```python
from build123d import *

# Parameters (mm, degrees)
DODANIE_WYCI_GNI_CIE1_DEPTH     = 3
SZKIC2_R                        = 1.35
WYTNIJ_WYCI_GNI_CIE1_DEPTH      = 3
DODANIE_WYCI_GNI_CIE2_DEPTH     = 40
WYTNIJ_WYCI_GNI_CIE4_DEPTH      = 65.691575959
WYTNIJ_WYCI_GNI_CIE4_DEPTH_BACK = 65.691575959
SZKIC6_R                        = 1.05
ZAOKR_GLENIE8_R                 = 20
ZAOKR_GLENIE9_R                 = 20
ZAOKR_GLENIE10_R                = 2
ZAOKR_GLENIE11_R                = 2


with BuildPart() as part:
    # Szkic1 → Dodanie-wyciągnięcie1 (new body)
    with BuildSketch(Plane(origin=(0, 0, 0), x_dir=(1, 0, 0), z_dir=(0, 1, 0))):
        with BuildLine():
            Line((-23.5, -20), (23.5, -20))
            ThreePointArc((23.5, -20), (24.560660172, -19.560660172), (25, -18.5))
            Line((25, -18.5), (25, 18.5))
            ThreePointArc((25, 18.5), (24.560660172, 19.560660172), (23.5, 20))
            Line((23.5, 20), (-23.5, 20))
            ThreePointArc((-23.5, 20), (-24.560660172, 19.560660172), (-25, 18.5))
            Line((-25, 18.5), (-25, -18.5))
            ThreePointArc((-25, -18.5), (-24.560660172, -19.560660172), (-23.5, -20))
        make_face()
    extrude(amount=DODANIE_WYCI_GNI_CIE1_DEPTH)

    # Szkic2 → Wytnij-wyciągnięcie1 (cut)
    with BuildSketch(Plane(origin=(0, 3, 0), x_dir=(1, 0, 0), z_dir=(0, 1, 0))):
        with Locations(Location((-22, 17, 0), (0, 0, 270))):
            Circle(SZKIC2_R)
        with Locations(Location((22, 17, 0), (0, 0, 270))):
            Circle(SZKIC2_R)
        with Locations(Location((-22, -17, 0), (0, 0, 270))):
            Circle(SZKIC2_R)
        with Locations(Location((22, -17, 0), (0, 0, 270))):
            Circle(SZKIC2_R)
        with BuildLine():
            Line((7.65, -3.086345678), (-7.65, -3.086345678))
            ThreePointArc((-7.65, -3.086345678), (-9.771320344, -2.207666021), (-10.65, -0.086345678))
            Line((-10.65, -0.086345678), (-10.65, 0.086345678))
            ThreePointArc((-10.65, 0.086345678), (-9.771320344, 2.207666021), (-7.65, 3.086345678))
            Line((-7.65, 3.086345678), (7.65, 3.086345678))
            ThreePointArc((7.65, 3.086345678), (9.771320344, 2.207666021), (10.65, 0.086345678))
            Line((10.65, 0.086345678), (10.65, -0.086345678))
            ThreePointArc((10.65, -0.086345678), (9.771320344, -2.207666021), (7.65, -3.086345678))
        make_face()
    extrude(amount=-WYTNIJ_WYCI_GNI_CIE1_DEPTH, mode=Mode.SUBTRACT)

    # Szkic3 → Dodanie-wyciągnięcie2 (add)
    with BuildSketch(Plane(origin=(0, 3, 0), x_dir=(1, 0, 0), z_dir=(0, 1, 0))):
        Polygon((-15.75, 6), (-12.5, 6), (-12.5, 14), (-19, 14), (-19, -20), (-15.75, -20), align=None)
        Polygon((15.75, 6), (15.75, -20), (19, -20), (19, 14), (12.5, 14), (12.5, 6), align=None)
    extrude(amount=DODANIE_WYCI_GNI_CIE2_DEPTH)

    # Szkic6 → Wytnij-wyciągnięcie4 (cut, two sides: drawn at the far end of the back side and taken through both)
    with BuildSketch(Plane.ZY.offset(19).offset(-WYTNIJ_WYCI_GNI_CIE4_DEPTH_BACK)):
        with Locations((-10, 20.5)):
            Circle(SZKIC6_R)
    extrude(amount=WYTNIJ_WYCI_GNI_CIE4_DEPTH + WYTNIJ_WYCI_GNI_CIE4_DEPTH_BACK, mode=Mode.SUBTRACT)

    # Zaokrąglenie8
    zaokr_glenie8_edges = [part.edges().sort_by_distance(p)[0] for p in [
        (-17.375, 43, 20),
    ]]
    fillet(zaokr_glenie8_edges, radius=ZAOKR_GLENIE8_R)

    # Zaokrąglenie9
    zaokr_glenie9_edges = [part.edges().sort_by_distance(p)[0] for p in [
        (17.375, 43, 20),
    ]]
    fillet(zaokr_glenie9_edges, radius=ZAOKR_GLENIE9_R)

    # Zaokrąglenie10
    zaokr_glenie10_edges = [part.edges().sort_by_distance(p)[0] for p in [
        (-15.75, 43, -14),
    ]]
    fillet(zaokr_glenie10_edges, radius=ZAOKR_GLENIE10_R)

    # Zaokrąglenie11
    zaokr_glenie11_edges = [part.edges().sort_by_distance(p)[0] for p in [
        (15.75, 43, -14),
    ]]
    fillet(zaokr_glenie11_edges, radius=ZAOKR_GLENIE11_R)


solid = part.part
```
Model file for the job. Use its own axes, mm. A direction names the side the tool comes from. Round coordinates to 2 decimals unless told otherwise and drop trailing zeros. Write each loop counter-clockwise with the first axis right and the second up, starting at its lowest first coordinate (ties: lowest second). Pieces come first, ordered by that corner, then holes. Notation, with made-up numbers: (17, 11) - (59, 11) arc R33 cw to (59, 50) - close; hole circle Ø9 at (13, 86.5). An arc over 180 degrees is marked (long way). Use CSV: the item, a comma, the result in double quotes. Start each with the question number.
Item 1: Tool access for faces 1 (the face through (14, 23, -6)), 2 (the face through (16, 22, -14)), 3 (the face through (-12.5, 23, -10)): list every direction of +Z, -Z, +X, -X, +Y, -Y with a clear straight run to the whole face (end or side of a thin tool).
Item 2: Pin check, flat tips, straight feed: P1, Ø1.6, axis at x = 22, z = 17, coming from the +Y side; P2, Ø3, axis at x = 19.5, y = 28.5, coming from the +Z side; P3, Ø2, axis at x = -14.5, y = 23, coming from the -Z side; P4, Ø4, axis at y = 24.5, z = -9.5, coming from the +X side. Stop position of each tip, or through.
Item 3: Band-saw the part on B-B (y = 20.5). Write the cut outline in (x, z), and give its area (3 significant figures).
Item 4: Drill centre lines: L1, parallel to X at y = 2, z = -17; L2, parallel to X at y = 38.5, z = -9.5; L3, parallel to X at y = 37, z = 7.5. Where is each one in solid material? Low to high. Write a range as [from, to].
Item 5: Band-saw the part on C-C (x = -3.5). Write the cut outline in (y, z).
Item 6: Band-saw the part on D-D (z = -17). Write the cut outline in (x, y).
Item 7: Band-saw the part on A-A (x = 22). Write the cut outline in (y, z), and give its area (3 significant figures).
Item 8: Two-plate mould, pull along Z, no slides. Class faces 4 (the face through (-2, 1, 20)), 5 (the face through (-9.795, 1.521, -2.184)), 6 (the face through (25, 1, 0)): released by +Z, released by -Z, zero draft, split by the parting line, or undercut.
Checked values:
1,face 1,"+Z, +Y"
1,face 2,"-Z, +X, -X, +Y"
1,face 3,"+Z, -Z, +Y"
2,P1,"passes through"
2,P2,"stops at z = 19.58"
2,P3,"stops at z = -14"
2,P4,"stops at x = 19"
3,outline,"(-19, -14) - (-12.5, -14) - (-12.5, -11.05) - (-19, -11.05) - close; (-19, -8.95) - (-12.5, -8.95) - (-12.5, -6) - (-15.75, -6) - (-15.75, 20) - (-19, 20) - close; (12.5, -14) - (19, -14) - (19, -11.05) - (12.5, -11.05) - close; (12.5, -8.95) - (19, -8.95) - (19, 20) - (15.75, 20) - (15.75, -6) - (12.5, -6) - close"
3,area,"246 mm²"
4,L1,"x = [-25, -23.35], [-20.65, 20.65], [23.35, 25]"
4,L2,"x = [-19, -12.5], [12.5, 19]"
4,L3,"x = [-19, -15.75], [15.75, 19]"
5,outline,"(0, -20) - (3, -20) - (3, -3.09) - (0, -3.09) - close; (0, 3.09) - (3, 3.09) - (3, 20) - (0, 20) - close"
6,outline,"(-25, 0) - (-23.35, 0) - (-23.35, 3) - (-25, 3) - close; (-20.65, 0) - (20.65, 0) - (20.65, 3) - (-20.65, 3) - close; (23.35, 0) - (25, 0) - (25, 3) - (23.35, 3) - close"
7,outline,"(0, -20) - (3, -20) - (3, -18.35) - (0, -18.35) - close; (0, -15.65) - (3, -15.65) - (3, 15.65) - (0, 15.65) - close; (0, 18.35) - (3, 18.35) - (3, 20) - (0, 20) - close"
7,area,"104 mm²"
8,face 4,"released by +Z"
8,face 5,"undercut"
8,face 6,"zero draft"
